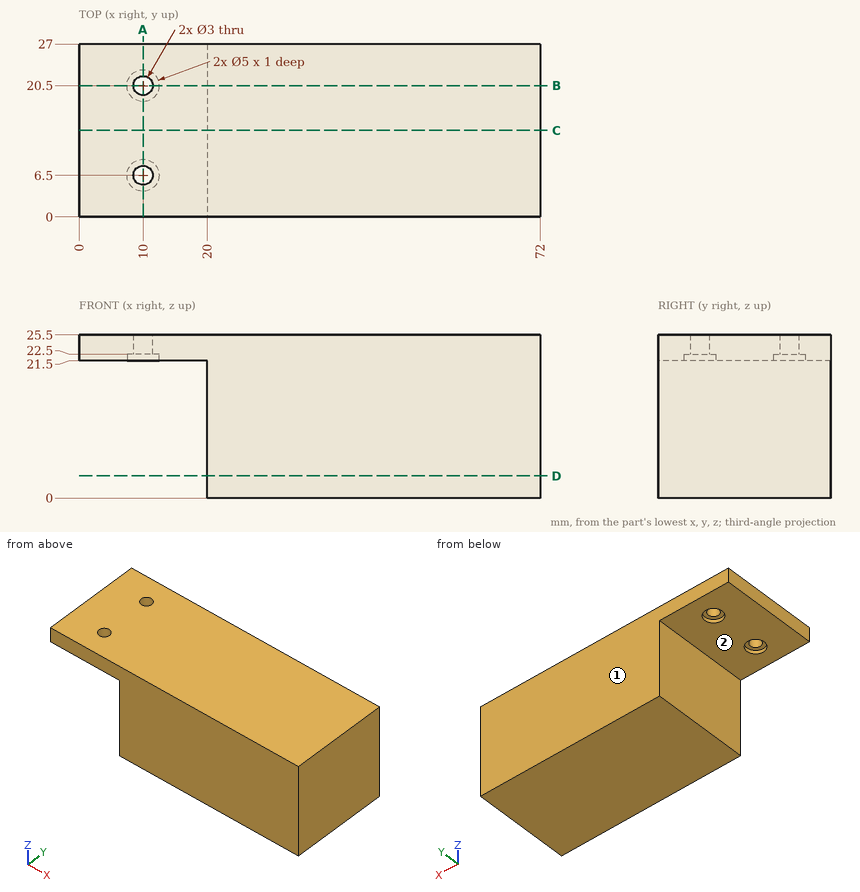
The drawing under review shows one solid part. Ordinate dimensions are in mm from its lowest x, y, z. A direction names the side the tool comes from. Coordinates: 2 decimals unless noted, no trailing zeros. Write each loop counter-clockwise with the first axis right and the second up, starting at its lowest first coordinate (ties: lowest second). Pieces come first, ordered by that corner, then holes. Notation, with made-up numbers: M 89,-22.75 L 129,-22.75 A31 cw 129,8.25 Z; hole C 68.25,67.5 d4. An arc over 180 degrees is marked long. Put each result on its own line as item: value.
1) Add section A-A on x = 10. Give the boundary of the cut face in (y, z), then the cut area to 3 significant figures.
Computed:
outline: M 0,21.5 L 4,21.5 L 4,22.5 L 5,22.5 L 5,25.5 L 0,25.5 Z; M 8,22.5 L 9,22.5 L 9,21.5 L 18,21.5 L 18,22.5 L 19,22.5 L 19,25.5 L 8,25.5 Z; M 22,22.5 L 23,22.5 L 23,21.5 L 27,21.5 L 27,25.5 L 22,25.5 Z
area: 80.0 mm2
2) Add section C-C on y = 13.5. Give the boundary of the cut face in (x, z).
Computed:
outline: M 0,21.5 L 20,21.5 L 20,0 L 72,0 L 72,25.5 L 0,25.5 Z
3) Add section D-D on z = 3.5. Give the boundary of the cut face in (x, y), then the cut area to 3 significant figures.
Computed:
outline: M 20,0 L 72,0 L 72,27 L 20,27 Z
area: 1,400 mm2
4) For the marked faces 1 and 2, list the 3-axis set-ups (+Z, -Z, +X, -X, +Y, -Y) from which the entire face can be reached by the end or side of a thin tool; tool diameter is ignored.
Computed:
face 1: +Z, -Z, +X, -X, +Y
face 2: -Z, -X, +Y, -Y
5) Add section B-B on y = 20.5. Give the boundary of the cut face in (x, z), then the cut area to 3 significant figures.
Computed:
outline: M 0,21.5 L 7.5,21.5 L 7.5,22.5 L 8.5,22.5 L 8.5,25.5 L 0,25.5 Z; M 11.5,22.5 L 12.5,22.5 L 12.5,21.5 L 20,21.5 L 20,0 L 72,0 L 72,25.5 L 11.5,25.5 Z
area: 1,390 mm2
6) Clearance check with flat-ended pins moving along their axes: pin 1 Ø2.5 at (x, y) = (10, 6.5) entering from -Z; pin 2 Ø3 at (y, z) = (24.5, 19.5) entering from -X; pin 3 Ø8 at (x, y) = (10, 6.5) entering from -Z; pin 4 Ø4 at (x, y) = (10, 20.5) entering from -Z. State where each tip first meets the part, or that it passes through.
Computed:
pin 1: passes through
pin 2: stops at x = 20
pin 3: stops at z = 21.5
pin 4: stops at z = 22.5
7) Wall thickness on probe 1 along Y at (x, z) = (10, 24.45); probe 2 along X at (y, z) = (6.5, 23.3); probe 3 along X at (y, z) = (6.5, 21.75): over which ranges is each line inside the solid? List them lowest first. Write a range as [from, to].
Computed:
probe 1: y = [0, 5], [8, 19], [22, 27]
probe 2: x = [0, 8.5], [11.5, 72]
probe 3: x = [0, 7.5], [12.5, 72]
